Source: three-view drawing plus pictorial views. Frame: mm from the lowest corner of the part. Give positions to 0.01 mm unless a question says otherwise; leave off trailing zeros. Write each loop counter-clockwise with the first axis right and the second up, starting at its lowest first coordinate (ties: lowest second). Pieces come first, ordered by that corner, then holes. Notation, with made-up numbers: (23.5, 25) -> (56.5, 25) arc R14 ccw to (56.5, 31) -> close; hole circle Ø7 at (74, -29.5). An arc over 180 degrees is marked (long way). Write item = value, one per line.
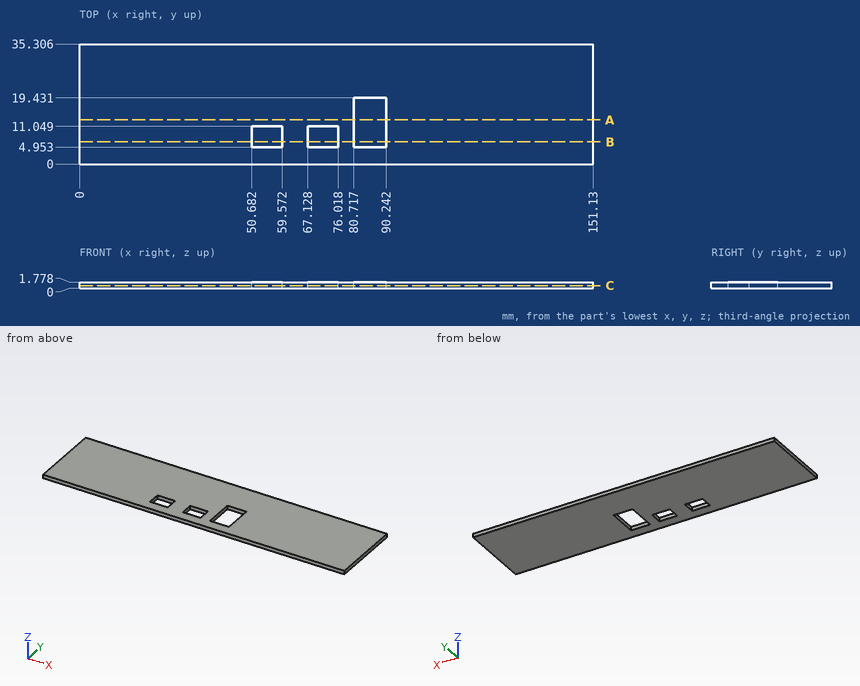
1) Material intervals for L1, parallel to X at y = 10, z = 1.5; L2, parallel to X at y = 16, z = 1.1; L3, parallel to Y at x = 85.5, z = 0.2, sorted ascending.
Computed:
L1 = 0 to 50.68, 59.57 to 67.13, 76.02 to 80.72, 90.24 to 151.13
L2 = 0 to 80.72, 90.24 to 151.13
L3 = 0 to 4.95, 19.43 to 35.31
2) Cut plane A-A (y = 13). Return the cut outline in (x, z).
Computed:
outline = (0, 0) -> (80.72, 0) -> (80.72, 1.78) -> (0, 1.78) -> close; (90.24, 0) -> (151.13, 0) -> (151.13, 1.78) -> (90.24, 1.78) -> close
3) Contact query for a flat-ended pin moving along its axis: pin 1 (0.9 mm diameter, centred on y = 8, z = 1, fed in from -X). Output: stop coordinate, or through.
Computed:
pin_1 = 0
4) Cut plane B-B (y = 6.5). Return the cut outline in (x, z), then the cut area to 3 significant figures.
Computed:
outline = (0, 0) -> (50.68, 0) -> (50.68, 1.78) -> (0, 1.78) -> close; (59.57, 0) -> (67.13, 0) -> (67.13, 1.78) -> (59.57, 1.78) -> close; (76.02, 0) -> (80.72, 0) -> (80.72, 1.78) -> (76.02, 1.78) -> close; (90.24, 0) -> (151.13, 0) -> (151.13, 1.78) -> (90.24, 1.78) -> close
area = 220 mm²
5) Cut plane C-C (z = 0.7). Return the cut outline in (x, y), then the cut area to 3 significant figures.
Computed:
outline = (0, 0) -> (151.13, 0) -> (151.13, 35.31) -> (0, 35.31) -> close; hole (50.68, 4.95) -> (59.57, 4.95) -> (59.57, 11.05) -> (50.68, 11.05) -> close; hole (67.13, 4.95) -> (76.02, 4.95) -> (76.02, 11.05) -> (67.13, 11.05) -> close; hole (80.72, 4.95) -> (90.24, 4.95) -> (90.24, 19.43) -> (80.72, 19.43) -> close
area = 5,090 mm²
